Solid Edge part; units mm, degrees
sketch "Sketch1" plane through (0, 0, 0) normal (0, 0, 1) x (1, 0, 0)
  circle A0 centre (0, 0) radius 9.525
extrude "Protrusion1" add sketch "Sketch1" against normal blind 45.72
sketch "Sketch2" plane through (0, 0, 0) normal (0, 0, 1) x (1, 0, 0)
  line L0 (8.9619, -15.5225) -> (17.9238, 0)
  line L1 (17.9238, 0) -> (8.9619, 15.5225)
  line L2 (8.9619, 15.5225) -> (-8.9619, 15.5225)
  line L3 (-8.9619, 15.5225) -> (-17.9238, 0)
  line L4 (-17.9238, 0) -> (-8.9619, -15.5225)
  line L5 (-8.9619, -15.5225) -> (8.9619, -15.5225)
extrude "ExtrudedProtrusion_2" add sketch "Sketch2" along normal blind 6.35
fillet "Round_1" radius 1.905 6 edges at (13.4429, -7.7612, 6.35) (0, -15.5225, 6.35) (-13.4429, -7.7612, 6.35) (-13.4429, 7.7612, 6.35) (0, 15.5225, 6.35) (13.4429, 7.7612, 6.35)
Could you check a few things on this model? Use its own coordinates, in mm. A direction names the side the tool comes from. Coordinates: 2 decimals unless noted, no trailing zeros. Loops run counter-clockwise (first coordinate to the right, second up) from the corner with the lowest first, then second, coordinate; pieces in that order, holes last.
1) Which directions (+Z, -Z, +X, -X, +Y, -Y) give clear straight access to the entire face, cutting with the end or side of a thin tool? Please do faces 1 (the face through (13.506, 7.653, 2.191)), 2 (the face through (8, 7, 0)).
Reported:
face 1: +Z, -Z, +X, +Y
face 2: -Z
2) Imagine slicing it at D-D (z = -30.5). List the corners of the cut face in (x, y) for me (3 decimals).
Reported:
outline: circle Ø19.05 at (0, 0)
3) Imagine slicing it at A-A (z = 2.5). List the corners of the cut face in (x, y) for me.
Reported:
outline: (-17.92, 0) - (-8.96, -15.52) - (8.96, -15.52) - (17.92, 0) - (8.96, 15.52) - (-8.96, 15.52) - close
4) Will these pins go through, and if not, where does the flat tip stop? pin 1 Ø4 at (x, z) = (-4.5, -16) entering from -Y; pin 2 Ø12 at (y, z) = (-8, -26.5) entering from +X; pin 3 Ø3 at (x, z) = (4.5, -18) entering from +Y; pin 4 Ø6 at (x, z) = (5, -0.5) entering from +Y.
Reported:
pin 1: stops at y = -9.19
pin 2: stops at x = 9.31
pin 3: stops at y = 9.04
pin 4: stops at y = 15.52
5) Please list where these lines run through material, in increasing order: line 1 along Z through (x, y) = (3, -12); line 2 along X through (y, z) = (0.5, -13); line 3 along Z through (x, y) = (-13, 5).
Reported:
line 1: z = 0 to 6.35
line 2: x = -9.51 to 9.51
line 3: z = 0 to 6.34
